```python
from build123d import *

# Parameters (mm, degrees)
SKETCH1_W           = 200
SKETCH1_H           = 120
BOSS_EXTRUDE1_DEPTH = 100
SHELL1_T            = -10
SKETCH2_R           = 30
BOSS_EXTRUDE2_DEPTH = 20
BOSS_EXTRUDE3_START = 20
SKETCH3_R           = 30
BOSS_EXTRUDE3_DEPTH = 20
SKETCH4_R           = 20
CUT_EXTRUDE1_DEPTH  = 35
CUT_EXTRUDE2_START  = -35
SKETCH5_R           = 20
CUT_EXTRUDE2_DEPTH  = 35
SKETCH7_R           = 4.5
CUT_EXTRUDE3_DEPTH  = 10
CUT_EXTRUDE4_START  = 10
SKETCH8_R           = 4.5
CUT_EXTRUDE4_DEPTH  = 10
FILLET1_R           = 2


with BuildPart() as part:
    # Sketch1 → Boss-Extrude1 (new body)
    with BuildSketch(Plane.XY):
        Rectangle(SKETCH1_W, SKETCH1_H)
    extrude(amount=BOSS_EXTRUDE1_DEPTH)

    # Shell1
    shell1_openings = [part.faces().sort_by_distance(p)[0] for p in [
        (0, 0, 100),
    ]]
    offset(amount=SHELL1_T, openings=shell1_openings, kind=Kind.INTERSECTION)

    # Sketch2 → Boss-Extrude2 (add)
    with BuildSketch(Plane(origin=(-75, 0, 0), x_dir=(0, 0, -1), z_dir=(1, 0, 0))):
        with Locations((0, 50)):
            Circle(SKETCH2_R)
    extrude(amount=-BOSS_EXTRUDE2_DEPTH)

    # Sketch3 → Boss-Extrude3 (add)
    with BuildSketch(Plane(origin=(75, 0, 0), x_dir=(0, 0, -1), z_dir=(1, 0, 0)).offset(BOSS_EXTRUDE3_START)):
        with Locations((0, 50)):
            Circle(SKETCH3_R)
    extrude(amount=-BOSS_EXTRUDE3_DEPTH)

    # Sketch4 → Cut-Extrude1 (cut)
    with BuildSketch(Plane(origin=(-95, 0, 0), x_dir=(0, 0, -1), z_dir=(1, 0, 0))):
        with Locations(Location((0, 50, 0), (0, 0, 150))):
            Circle(SKETCH4_R)
    extrude(amount=CUT_EXTRUDE1_DEPTH, mode=Mode.SUBTRACT)

    # Sketch5 → Cut-Extrude2 (cut)
    with BuildSketch(Plane(origin=(95, 0, 0), x_dir=(0, 0, -1), z_dir=(1, 0, 0)).offset(CUT_EXTRUDE2_START)):
        with Locations(Location((0, 50, 0), (0, 0, 150))):
            Circle(SKETCH5_R)
    extrude(amount=CUT_EXTRUDE2_DEPTH, mode=Mode.SUBTRACT)

    # Sketch7 → Cut-Extrude3 (cut)
    with BuildSketch(Plane.XY.offset(100)):
        with Locations((95, 55)):
            Circle(SKETCH7_R)
        with Locations((95, -55)):
            Circle(SKETCH7_R)
        with Locations((-95, 55)):
            Circle(SKETCH7_R)
        with Locations((-95, -55)):
            Circle(SKETCH7_R)
    extrude(amount=-CUT_EXTRUDE3_DEPTH, mode=Mode.SUBTRACT)

    # Sketch8 → Cut-Extrude4 (cut)
    with BuildSketch(Plane.XY.offset(CUT_EXTRUDE4_START)):
        with Locations((95, 55)):
            Circle(SKETCH8_R)
        with Locations((95, -55)):
            Circle(SKETCH8_R)
        with Locations((-95, 55)):
            Circle(SKETCH8_R)
        with Locations((-95, -55)):
            Circle(SKETCH8_R)
    extrude(amount=-CUT_EXTRUDE4_DEPTH, mode=Mode.SUBTRACT)

    # Fillet1
    fillet1_edges = [part.edges().sort_by_distance(p)[0] for p in [
        (100, -60, 50),
        (-100, -60, 50),
        (-100, 60, 50),
        (100, 60, 50),
    ]]
    fillet(fillet1_edges, radius=FILLET1_R)


solid = part.part
```
The listing builds one solid part. Answer for the finished solid, in the listing's coordinates (mm). A direction names the side the tool comes from. Coordinates: 2 decimals unless noted, no trailing zeros. Loops run counter-clockwise (first coordinate to the right, second up) from the corner with the lowest first, then second, coordinate; pieces in that order, holes last. Notation, with made-up numbers: (81, 56.25) -> (140, 56.25) arc R26 cw to (140, 88.25) -> close; hole circle Ø5 at (-7, 44.25). An arc over 180 degrees is marked (long way). Return JSON: item names as keys, results as strings. Group by question number.
(1) Find the intervals of material crossed by probe 1 along Y at (x, z) = (-95, 94); probe 2 along Y at (x, z) = (43, 71.5); probe 3 along X at (y, z) = (31, 56), in increasing order. Write a range as from..to.
(2) Determine the mould class of faces 1 (the flat face through (-1, 50, 54)), 2 (the cylindrical face through (85.14, 66.563, -25.013)), 3 (the flat face through (-1, 1, 0)) for opening direction Y: released by +Y, released by -Y, zero draft, split by the parting line, or undercut.
(3) A cutting plane is placed at C-C on y = -55. Write down the section's boundary in (x, z), and give its area (3 significant figures).
(4) A cutting plane is placed at B-B on x = 26.5. Write down the section's boundary in (y, z).
(5) A cutting plane is placed at D-D on z = 92.5. Write down the section's boundary in (x, y).
(6) A cutting plane is placed at A-A on z = 76. Write down the section's boundary in (x, y).
(7) Given pin 1 Ø1.3 at (x, y) = (98, 55.5) entering from -Z; pin 2 Ø11.5 at (x, y) = (-95, -55) entering from -Z; pin 3 Ø1 at (x, y) = (-37.5, -40) entering from +Z, each flat-ended and moving along its own axis, determine where each tip first touches the part or whether it passes through.
(8) Which of the six approach directions +Z, -Z, +X, -X, +Y, -Y give full straight-line access (tool end or side, diameter ignored) to faces 4 (the flat face through (-95, 55, 90)), 5 (the flat face through (95, 45, 9)), 6 (the flat face through (-97, 55, 10)), 7 (the flat face through (75, 63, -16))?
The answers:
{
 "1": {"probe 1": "y = -60..-59.5, -50.5..50.5, 59.5..60", "probe 2": "y = -60..-50, 50..60", "probe 3": "x = -100..-90, 90..100"},
 "2": {"face 1": "undercut", "face 2": "split by the parting line", "face 3": "zero draft"},
 "3": {"outline": "(-100, 0) -> (-99.5, 0) -> (-99.5, 10) -> (-90.5, 10) -> (-90.5, 0) -> (90.5, 0) -> (90.5, 10) -> (99.5, 10) -> (99.5, 0) -> (100, 0) -> (100, 100) -> (99.5, 100) -> (99.5, 90) -> (90.5, 90) -> (90.5, 100) -> (-90.5, 100) -> (-90.5, 90) -> (-99.5, 90) -> (-99.5, 100) -> (-100, 100) -> close", "area": "19,600 mm^2"},
 "4": {"outline": "(-60, 0) -> (60, 0) -> (60, 100) -> (50, 100) -> (50, 10) -> (-50, 10) -> (-50, 100) -> (-60, 100) -> close"},
 "5": {"outline": "(-100, -58) arc R2 ccw to (-98, -60) -> (98, -60) arc R2 ccw to (100, -58) -> (100, 58) arc R2 ccw to (98, 60) -> (-98, 60) arc R2 ccw to (-100, 58) -> close; hole circle Ø9 at (-95, -55); hole circle Ø9 at (-95, 55); hole (-90, -50) -> (90, -50) -> (90, 50) -> (-90, 50) -> close; hole circle Ø9 at (95, -55); hole circle Ø9 at (95, 55)"},
 "6": {"outline": "(-100, -58) arc R2 ccw to (-98, -60) -> (98, -60) arc R2 ccw to (100, -58) -> (100, 58) arc R2 ccw to (98, 60) -> (-98, 60) arc R2 ccw to (-100, 58) -> close; hole (-90, -50) -> (90, -50) -> (90, 50) -> (-90, 50) -> close"},
 "7": {"pin 1": "stops at z = 10", "pin 2": "stops at z = 0", "pin 3": "stops at z = 10"},
 "8": {"face 4": "+Z", "face 5": "none", "face 6": "-Z", "face 7": "-Z, +Y"}
}
